from build123d import *

# Parameters (mm, degrees)
SKETCH1_R           = 1.125
BOSS_EXTRUDE5_DEPTH = 8.5
SKETCH3_W           = 15.998285444
SKETCH3_H           = 4.5
SKETCH3_W_2         = 14.781977404
CUT_EXTRUDE1_DEPTH  = 8.5


with BuildPart() as part:
    # Sketch1 → Boss-Extrude5 (new body)
    with BuildSketch(Plane(origin=(0, 0, 0), x_dir=(1, 0, 0), z_dir=(0, 1, 0))):
        with BuildLine():
            Line((-27.093662294, 63.483418595), (-14.330111131, 42.417509095))
            ThreePointArc((-14.330111131, 42.417509095), (-8.606773323, 42.92644123), (-12.512429784, 47.140875379))
            Line((-12.512429784, 47.140875379), (-22.065450081, 62.90788712))
            ThreePointArc((-22.065450081, 62.90788712), (-23.992920625, 68.320877504), (-27.093662294, 63.483418595))
        make_face()
        with Locations(Location((-24.356818103, 65.141635672, 0), (0, 0, 270))):
            Circle(SKETCH1_R, mode=Mode.SUBTRACT)
        with Locations(Location((-11.59326694, 44.075726171, 0), (0, 0, 270))):
            Circle(SKETCH1_R, mode=Mode.SUBTRACT)
    extrude(amount=BOSS_EXTRUDE5_DEPTH)

    # Sketch3 → Cut-Extrude1 (cut)
    with BuildSketch(Plane(origin=(8.31694784, 0, -5.039126807), x_dir=(0.518192836351311, 0, 0.855263809800335), z_dir=(-0.8552638098003349, 0, 0.5181928363513109))):
        with Locations((-69.33395488, 4.25)):
            Rectangle(SKETCH3_W, SKETCH3_H)
        with Locations((-43.312932661, 4.25)):
            Rectangle(SKETCH3_W_2, SKETCH3_H)
    extrude(amount=-CUT_EXTRUDE1_DEPTH, mode=Mode.SUBTRACT)


solid = part.part
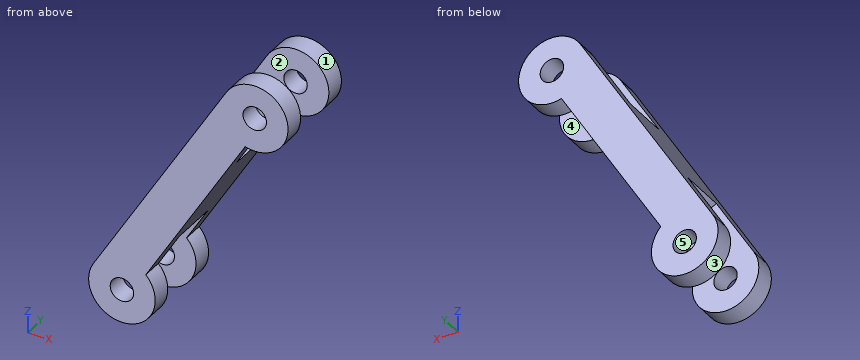
Work out the finished part from the listing and answer in its coordinate system (mm). Face numbers are marked on the shaded views. A direction names the side the tool comes from. Round coordinates to 2 decimals unless told otherwise and drop trailing zeros. Loops run counter-clockwise (first coordinate to the right, second up) from the corner with the lowest first, then second, coordinate; pieces in that order, holes last. Notation, with made-up numbers: (36, -6) - (51, -6) arc R22 ccw to (51, 9) - close; hole circle Ø5 at (24.25, 13). An arc over 180 degrees is marked (long way). One line per item, written item: value.
Q1. Find section D-D on z = -46.5. Give the vertices of the cut face in (x, y).
Check values:
outline: (-16.8, 0) - (-9.5, 0) - (-9.5, 2) - (-16.8, 2) - close; (-16.8, 6.5) - (-9.5, 6.5) - (-9.5, 8.5) - (-16.8, 8.5) - close
Q2. The mould has two halves that part along X. Classify the marked faces 3, 4 and 5: +X half, -X half, draft (parallel to the pull), parting line (faces both ways), or undercut.
Check values:
face 3: parting line
face 4: draft
face 5: undercut
Q3. Straight lines are drawn through the part: probe 1 along Y at (x, z) = (-25.75, -66.5); probe 2 along Z at (x, y) = (-21.5, 7.5); probe 3 along X at (y, z) = (8, -53). For each, find the intervals that lie inside material, in ascending order.
Check values:
probe 1: 0 to 2, 6.5 to 8.5
probe 2: -66.58 to -63.7, -61.97 to -54.25
probe 3: -20.74 to -16.06
Q4. For the marked faces 1 and 2, determine the directions among +Z, -Z, +X, -X, +Y, -Y from which every point of the face is accessible in a straight line to the end or side of a thin tool.
Check values:
face 1: +Y, -Y
face 2: +Z, +X
Q5. Find section C-C on y = 7.5. State how many separate pieces and enclosed holes the cut face has, and give its area (3 significant figures).
Check values:
separate pieces: 1
enclosed holes: 2
area: 134 mm2
Q6. Each of these flat-tipped pins is pushed along its axis until it touches: pin 1 Ø1 at (x, y) = (-18, 2) entering from +Z; pin 2 Ø1 at (x, y) = (-12, 1.5) entering from -Z; pin 3 Ø6 at (x, z) = (-22.5, -61) entering from -Y; pin 4 Ø5 at (y, z) = (7, -52.5) entering from +X. Where does it stop, or does it pass through?
Check values:
pin 1: z = -47.65
pin 2: z = -47.28
pin 3: y = 0
pin 4: x = -14.24
Q7. Find section B-B on x = -13.75. Give the vertices of the cut face in (y, z).
Check values:
outline: (0, -49.18) - (2, -49.18) - (2, -41.71) - (0, -41.71) - close; (6.5, -49.18) - (8.5, -49.18) - (8.5, -41.71) - (6.5, -41.71) - close
Q8. Find section A-A on z = -64.5. Give the vertices of the cut face in (x, y).
Check values:
outline: (-27.49, 0) - (-25.28, 0) - (-25.28, 2) - (-27.49, 2) - close; (-27.49, 6.5) - (-25.28, 6.5) - (-25.28, 8.5) - (-27.49, 8.5) - close; (-23.43, 0) - (-21.22, 0) - (-21.22, 2) - (-23.43, 2) - close; (-23.43, 6.5) - (-21.22, 6.5) - (-21.22, 8.5) - (-23.43, 8.5) - close
